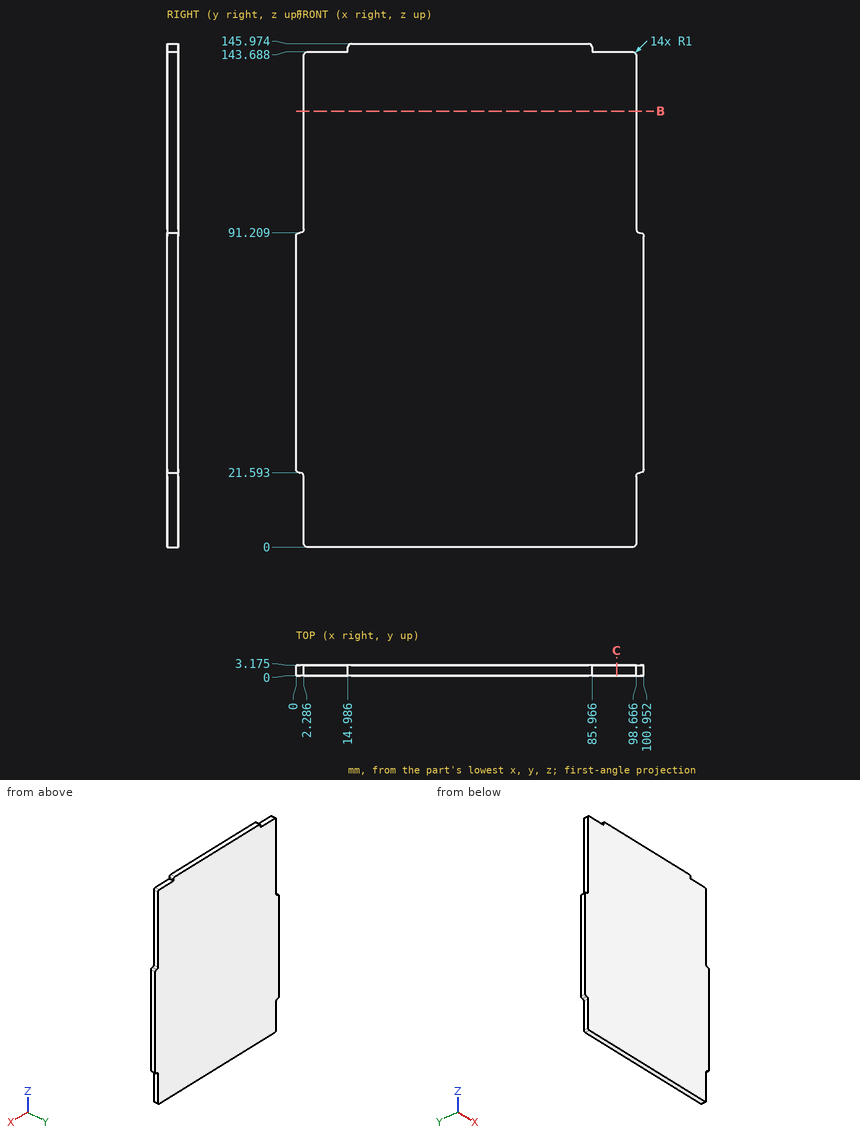
Source: three-view drawing plus pictorial views. Frame: mm from the lowest corner of the part. Coordinates: 2 decimals unless noted, no trailing zeros. Loops run counter-clockwise (first coordinate to the right, second up) from the corner with the lowest first, then second, coordinate; pieces in that order, holes last. Notation, with made-up numbers: (-9.75, 15.25) -> (34.25, 15.25) arc R4 ccw to (34.25, 22.25) -> close; hole circle Ø6 at (-2.5, -21). An arc over 180 degrees is marked (long way). Write each question's results on one line, items separated by ' | '. Start each with the question number.
Q1. Section C-C, the plane x = 93. Return the cut outline in (y, z) (1 decimal).
Q2. Section B-B, the plane z = 126.5. Return the cut outline in (x, y) (1 decimal).
Q3. Ray query, line 1 (X direction, y = 2.65, z = 14); line 2 (Z direction, x = 91.5, y = 0.55); line 3 (X direction, y = 1.45, z = 90.5). Return the intervals inside material, ascending. Write a range as from..to.
Q4. Pin query (flat end, axial travel): pin 1 (0.6 mm diameter, centred on y = 1.5, z = 144.5, fed in from +X); pin 2 (1 mm diameter, centred on y = 1.5, z = 14, fed in from -X). Return the tip coordinate at first contact, or that it passes through.
Found:
1) outline: (0, 0) -> (3.2, 0) -> (3.2, 143.7) -> (0, 143.7) -> close
2) outline: (2.3, 0) -> (98.7, 0) -> (98.7, 3.2) -> (2.3, 3.2) -> close
3) line 1: 2.29..98.67 | line 2: 0..143.69 | line 3: 0.04..100.91
4) pin 1: x = 85.97 | pin 2: x = 2.29
